Autodesk Inventor part; units mm, degrees
ref_plane "YZ Plane" through (0, 0, 0) normal (1, 0, 0) x (0, 1, 0)
ref_plane "XZ Plane" through (0, 0, 0) normal (0, 1, 0) x (-1, 0, 0)
ref_plane "XY Plane" through (0, 0, 0) normal (0, 0, 1) x (1, 0, 0)
sketch "草圖1" plane through (0, 0, 0) normal (0, 1, 0) x (-1, 0, 0)
  line L0 (0, 0) -> (-70, 0)
  line L1 (-70, 0) -> (-70, 40)
  line L2 (-70, 40) -> (0, 40)
  line L3 (0, 40) -> (0, 0)
  dimension "d0" = 70
  dimension "d1" = 40
extrude "擠出1" add sketch "草圖1" along normal blind 40
sketch "草圖2" plane through (0, 0, 40) normal (0, 0, 1) x (1, 0, 0)
  line L0 (0, 0) -> (0, 40)
  line L1 (0, 40) -> (70, 40)
  line L2 (70, 40) -> (70, 0)
  line L3 (70, 0) -> (0, 0)
  line L4 (70, 40) -> (0, 40)
  line L5 (40, 40) -> (70, 40)
  line L6 (70, 40) -> (70, 10)
  line L7 (70, 10) -> (40, 10)
  line L8 (40, 10) -> (40, 40)
  dimension "d4" = 10
  dimension "d5" = 30
extrude "擠出2" cut sketch "草圖2" against normal blind 30 contours L1 L2 L7 L8
sketch "草圖3" plane through (0, 0, 10) normal (0, 0, 1) x (1, 0, 0)
  line L0 (40, 40) -> (40, 10)
  line L1 (40, 10) -> (70, 10)
  line L2 (70, 40) -> (70, 10)
  line L3 (40, 40) -> (70, 40)
  line L4 (0, 40) -> (40, 40)
  line L5 (0, 0) -> (0, 40)
  line L6 (70, 0) -> (0, 0)
  line L7 (70, 10) -> (70, 0)
  line L8 (40, 40) -> (70, 40)
  line L9 (70, 40) -> (70, 30)
  line L10 (70, 30) -> (40, 30)
  line L11 (40, 30) -> (40, 40)
  point P0 (40, 30)
  dimension "d8" = 10
extrude "擠出3" cut sketch "草圖3" against normal blind 10 contours L3 L2 L10 L0
sketch "草圖4" plane through (40, 10, 40) normal (1, 0, 0) x (0, 0, -1)
  line L0 (0, 0) -> (30, 0)
  line L1 (30, 0) -> (30, 20)
  line L2 (30, 20) -> (40, 20)
  line L3 (40, 30) -> (40, 20)
  line L4 (0, 30) -> (40, 30)
  line L5 (0, 0) -> (0, 30)
  line L6 (0, -10) -> (0, 0)
  line L7 (40, -10) -> (0, -10)
  line L8 (40, 20) -> (40, -10)
  line L9 (0, 0) -> (20, 30)
  dimension "d11" = 20
extrude "擠出4" cut sketch "草圖4" against normal through all contours L5 L4 L9
sketch "草圖5" plane through (70, 0, 0) normal (0, 0, -1) x (-1, 0, 0)
  line L0 (0, 30) -> (30, 30)
  line L1 (30, 30) -> (30, 40)
  line L2 (30, 40) -> (70, 40)
  line L3 (70, 40) -> (70, 0)
  line L4 (70, 0) -> (0, 0)
  line L5 (0, 0) -> (0, 30)
  line L6 (40, 40) -> (60, 40)
  line L7 (60, 40) -> (60, 20)
  line L8 (60, 20) -> (40, 20)
  line L9 (40, 20) -> (40, 40)
  line L10 (30, 40) -> (70, 40)
  point P0 (50, 40)
  dimension "d14" = 20
  dimension "d15" = 20
extrude "擠出5" cut sketch "草圖5" against normal through all contours L2 L7 L8 L9
fillet "圓角1" radius 20 1 edges at (70, 30, 5)
sketch "草圖6" plane through (40, 10, 40) normal (0, 1, 0) x (1, 0, 0)
  line L0 (0, 0) -> (-40, 0)
  line L1 (-40, 0) -> (-40, 40)
  line L2 (-40, 40) -> (30, 40)
  line L3 (30, 40) -> (30, 30)
  line L4 (30, 30) -> (0, 30)
  line L5 (0, 30) -> (0, 0)
  line L6 (30, 0) -> (0, 0)
  line L7 (30, 30) -> (30, 0)
  circle A0 centre (15, 15) radius 5
  dimension "d19" = 10
  dimension "d20" = 15
  dimension "d21" = 15
extrude "擠出6" cut sketch "草圖6" against normal through all contours A0
properties part number "31" material "鋼、碳鋼"
Here's how the part is built. I have some questions about the finished solid (model axes, mm). A direction names the side the tool comes from. Give positions to 0.01 mm unless a question says otherwise; leave off trailing zeros. Order: outer loops, then holes, each group sorted by start corner. A loop starts at its lowest first (then second) coordinate and runs counter-clockwise, first axis right, second up. Notation, with made-up numbers: M 47.5,29.5 L 55.5,29.5 A4 ccw 55.5,34.5 Z; hole C 64.25,65 d8. An arc over 180 degrees is marked long. Answer as a JSON object with one key per item and string values. Group by question number.
1) Please list where these lines run through material, in increasing order: L1, parallel to X at y = 24, z = 20; L2, parallel to X at y = 7, z = 25; L3, parallel to Z at x = 55, y = 6. Write a range as [from, to].
2) On a 3-axis mill with a long thin cutter (end or side, diameter ignored), from which of +Z, -Z, +X, -X, +Y, -Y can I reach the whole of each face in a straight line? I mean faces 4 (the flat face through (55, 20, 10)), 5 (the flat face through (20.3, 18.1, 34.6)), 6 (the flat face through (45, 30, 5)), 7 (the flat face through (35, 40, 10)), 8 (the flat face through (30, 30, 13)). Say none if no direction works.
3) Suppose I cut it at D-D, the plane z = 12. Write out the boundary of the cut face in (x, y).
4) Suppose I cut it at C-C, the plane x = 55. Write out the boundary of the cut face in (y, z), plus the area to 3 significant figures.
5) Suppose I cut it at A-A, the plane y = 34. Write out the boundary of the cut face in (x, z), plus the area to 3 significant figures.
6) Suppose I cut it at B-B, the plane z = 21. Write out the boundary of the cut face in (x, y).
7) I'm going to push flat-ended pins straight in: pin 1 Ø24 at (y, z) = (26, 24.5) entering from +X; pin 2 Ø16 at (x, z) = (20.5, 18.5) entering from +Y; pin 3 Ø1 at (x, y) = (38, 35.5) entering from +Z. Where does each tip first touch, or does it pass through?
8) We'd pull the mould along X, two halves only. Please class faces 1 (the flat face through (70, 5, 20)), 2 (the flat face through (59, 10, 29)), 3 (the cylindrical face through (53.92, 5.07, 29.88)): pulls with the +X half, pulls with the -X half, needs draft (parallel to the pull), parting line crosses it, or undercut.
Results found:
{
 "1": {"L1": "[0, 10], [30, 40]", "L2": "[0, 50], [60, 70]", "L3": "[0, 20], [30, 40]"},
 "2": {"face 4": "+Z, +X, +Y", "face 5": "+Z, +X, -X, +Y", "face 6": "+Z, -Z, +X, +Y", "face 7": "+Z, -Z, +X, -X, +Y", "face 8": "+Z, -Z, +Y"},
 "3": {"outline": "M 0,0 L 70,0 L 70,10 L 40,10 L 40,40 L 30,40 L 30,20 L 10,20 L 10,40 L 0,40 Z"},
 "4": {"outline": "M 0,0 L 29.36,0 L 29.36,10 L 10,10 L 10,20 L 0,20 Z; M 0,30 L 10,30 L 10,40 L 0,40 Z", "area": "494 mm²"},
 "5": {"outline": "M 0,0 L 10,0 L 10,24 L 0,24 Z; M 30,0 L 40,0 L 40,24 L 30,24 Z", "area": "480 mm²"},
 "6": {"outline": "M 0,0 L 52,0 L 52,10 L 40,10 L 40,38.5 L 30,38.5 L 30,20 L 10,20 L 10,38.5 L 0,38.5 Z; M 58,0 L 70,0 L 70,10 L 58,10 Z"},
 "7": {"pin 1": "x = 40", "pin 2": "y = 20", "pin 3": "z = 23.33"},
 "8": {"face 1": "pulls with the +X half", "face 2": "needs draft", "face 3": "undercut"}
}
